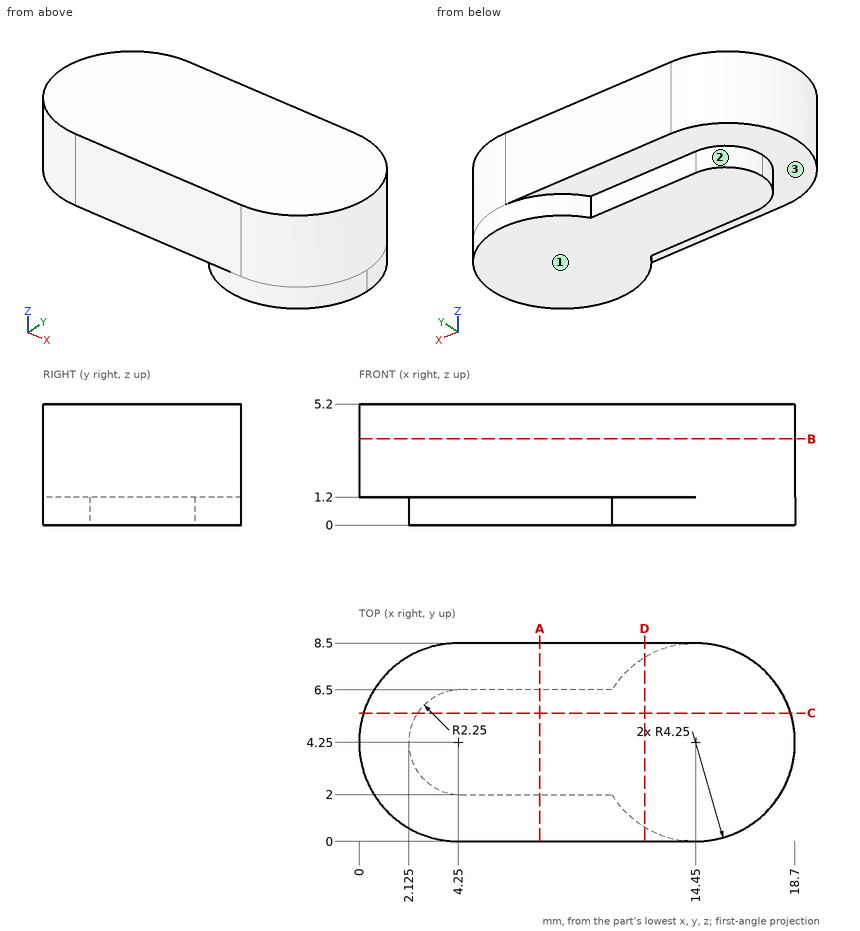
Answer from the drawing. Dimensions are ordinates in mm from the lowest x, y and z of the part. A direction names the side the tool comes from. Give positions to 0.01 mm unless a question says otherwise; leave off trailing zeros. Order: outer loops, then holes, each group sorted by start corner. A loop starts at its lowest first (then second) coordinate and runs counter-clockwise, first axis right, second up. Notation, with made-up numbers: (59, -7.5) - (66, -7.5) arc R19 cw to (66, 16.5) - close; hole circle Ø11 at (16, 28.25). An arc over 180 degrees is marked (long way). One line per item, written item: value. Start each with the question number.
1) A cutting plane is placed at D-D on x = 12.25. Give the vertices of the cut face in (y, z), then the cut area to 3 significant figures.
2) Find the intervals of material crossed by L1, parallel to Z at x = 6, y = 1.5; L2, parallel to X at y = 2.25, z = 4.55; L3, parallel to Y at x = 17.5, z = 2.15, in increasing order.
3) A tool of negligible diameter and unlimited length cuts with its end or side. For the marked faces 1, 2 and 3, from which of +Z, -Z, +X, -X, +Y, -Y can it reach the whole face along a straight path? Write none if from no direction.
4) Given pin 1 Ø3 at (x, z) = (16.5, 4.5) entering from +Y; pin 2 Ø1.5 at (y, z) = (1.5, 2) entering from -X; pin 3 Ø0.6 at (x, z) = (7, 0.5) entering from +Y, each flat-ended and moving along its own axis, determine where each tip first touches the part or whether it passes through.
5) A cutting plane is placed at B-B on z = 3.7. Give the vertices of the cut face in (x, y).
6) A cutting plane is placed at A-A on x = 7.75. Give the vertices of the cut face in (y, z), then the cut area to 3 significant figures.
7) A cutting plane is placed at C-C on y = 5.5. Give the vertices of the cut face in (x, z), then the cut area to 3 significant figures.
Answer sheet:
1. outline: (0, 1.2) - (0.61, 1.2) - (0.61, 0) - (7.89, 0) - (7.89, 1.2) - (8.5, 1.2) - (8.5, 5.2) - (0, 5.2) - close
1. area: 42.7 mm2
2. L1: z = 1.2 to 5.2
2. L2: x = 0.5 to 18.2
2. L3: y = 1.29 to 7.21
3. face 1: -Z, +X, -X, +Y, -Y
3. face 2: -Z, -X, +Y
3. face 3: -Z, -X, -Y
4. pin 1: stops at y = 8.46
4. pin 2: stops at x = 0.5
4. pin 3: stops at y = 6.5
5. outline: (4.25, 0) - (14.45, 0) arc R4.25 ccw to (14.45, 8.5) - (4.25, 8.5) arc R4.25 ccw to start
6. outline: (0, 1.2) - (2, 1.2) - (2, 0) - (6.5, 0) - (6.5, 1.2) - (8.5, 1.2) - (8.5, 5.2) - (0, 5.2) - close
6. area: 39.4 mm2
7. outline: (0.19, 1.2) - (2.5, 1.2) - (2.5, 0) - (18.51, 0) - (18.51, 5.2) - (0.19, 5.2) - close
7. area: 92.5 mm2
